For this review, take the finished solid that the model builds, in its own axes (mm). Face numbers are marked on the shaded views. Give positions to 0.01 mm unless a question says otherwise; leave off trailing zeros. Write each loop counter-clockwise with the first axis right and the second up, starting at its lowest first coordinate (ties: lowest second). Pieces come first, ordered by that corner, then holes.
Q1. Mouldability with a two-part tool opening along Z and no side actions: class the marked faces 1, 2, 3 and 4 as released by +Z, released by -Z, zero draft, split by the parting line, or undercut.
Q2. For line 1 (X direction, y = -0.9, z = 0); line 2 (X direction, y = -0.95, z = 2.5); line 3 (Z direction, x = 3, y = 0.6), list the stretches that pass through material, from the lowest coordinate up.
Q3. We need section B-B (z = 0). Write out the cut boundary in (x, y).
Q4. We need section D-D (x = -2). Write out the cut boundary in (y, z), then the cut area to 3 significant figures.
Q5. We need section C-C (x = 6). Write out the cut boundary in (y, z).
Q6. We need section A-A (y = 1.6). Write out the cut boundary in (x, z).
Q7. Insertion check: P1, Ø1.5, axis at x = 10, y = -1.5, coming from the +Z side. The pin has a flat end and moves straight along its axis. Give the tip position at first contact, or say it passes through.
```python
from build123d import *

# Parameters (mm, degrees)
SKETCH1_R             = 14.5
SKETCH1_R_2           = 6.65
SKETCH1_R_3           = 5.15
DISCO_SEPARADOR_DEPTH = 4
SKETCH2_W             = 7
SKETCH2_H             = 10
PATA_AL_HUESO_DEPTH   = 4


with BuildPart() as part:
    # Sketch1 → Disco_separador (new body)
    with BuildSketch(Plane(origin=(0, -2, 0), x_dir=(1, 0, 0), z_dir=(0, 1, 0))):
        with Locations(Location((0, 0, 0), (0, 0, 270))):
            Circle(SKETCH1_R)
        with Locations(Location((-5.5, 0, 0), (0, 0, 270))):
            Circle(SKETCH1_R_2, mode=Mode.SUBTRACT)
        with Locations(Location((5.5, -6.5, 0), (0, 0, 270))):
            Circle(SKETCH1_R_3, mode=Mode.SUBTRACT)
        with Locations(Location((5.5, 6.5, 0), (0, 0, 270))):
            Circle(SKETCH1_R_3, mode=Mode.SUBTRACT)
    extrude(amount=DISCO_SEPARADOR_DEPTH)

    # Sketch2 → Pata_al_hueso (add)
    with BuildSketch(Plane(origin=(0, -2, 0), x_dir=(1, 0, 0), z_dir=(0, 1, 0))):
        with Locations((-16, 0)):
            Rectangle(SKETCH2_W, SKETCH2_H)
    extrude(amount=PATA_AL_HUESO_DEPTH)


solid = part.part
```
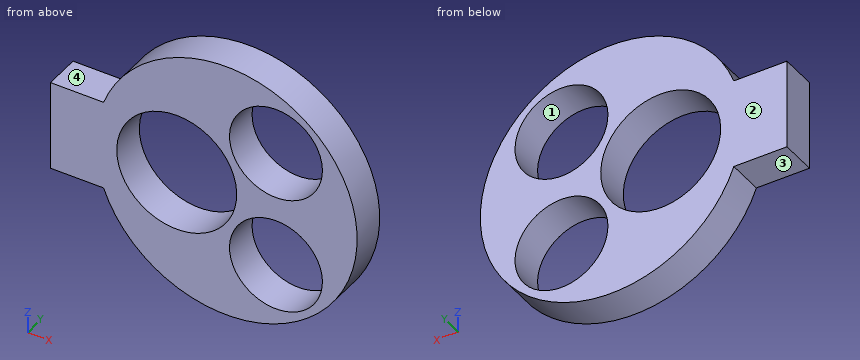
Computed:
1. face 1: undercut
1. face 2: zero draft
1. face 3: released by -Z
1. face 4: released by +Z
2. line 1: x = -19.5 to -12.15, 1.15 to 14.5
2. line 2: x = -19.5 to -11.66, 0.66 to 2.26, 8.74 to 14.28
2. line 3: z = -14.19 to -11, -2 to 2, 11 to 14.19
3. outline: (-19.5, -2) - (-12.15, -2) - (-12.15, 2) - (-19.5, 2) - close; (1.15, -2) - (14.5, -2) - (14.5, 2) - (1.15, 2) - close
4. outline: (-2, -14.36) - (2, -14.36) - (2, -5.65) - (-2, -5.65) - close; (-2, 5.65) - (2, 5.65) - (2, 14.36) - (-2, 14.36) - close
4. area: 69.7 mm2
5. outline: (-2, -13.2) - (2, -13.2) - (2, -11.63) - (-2, -11.63) - close; (-2, -1.37) - (2, -1.37) - (2, 1.37) - (-2, 1.37) - close; (-2, 11.63) - (2, 11.63) - (2, 13.2) - (-2, 13.2) - close
6. outline: (-19.5, -5) - (-13.61, -5) arc R14.5 ccw (long way) to (-13.61, 5) - (-19.5, 5) - close; hole circle Ø13.3 at (-5.5, 0); hole circle Ø10.3 at (5.5, -6.5); hole circle Ø10.3 at (5.5, 6.5)
7. P1: stops at z = 11.17
